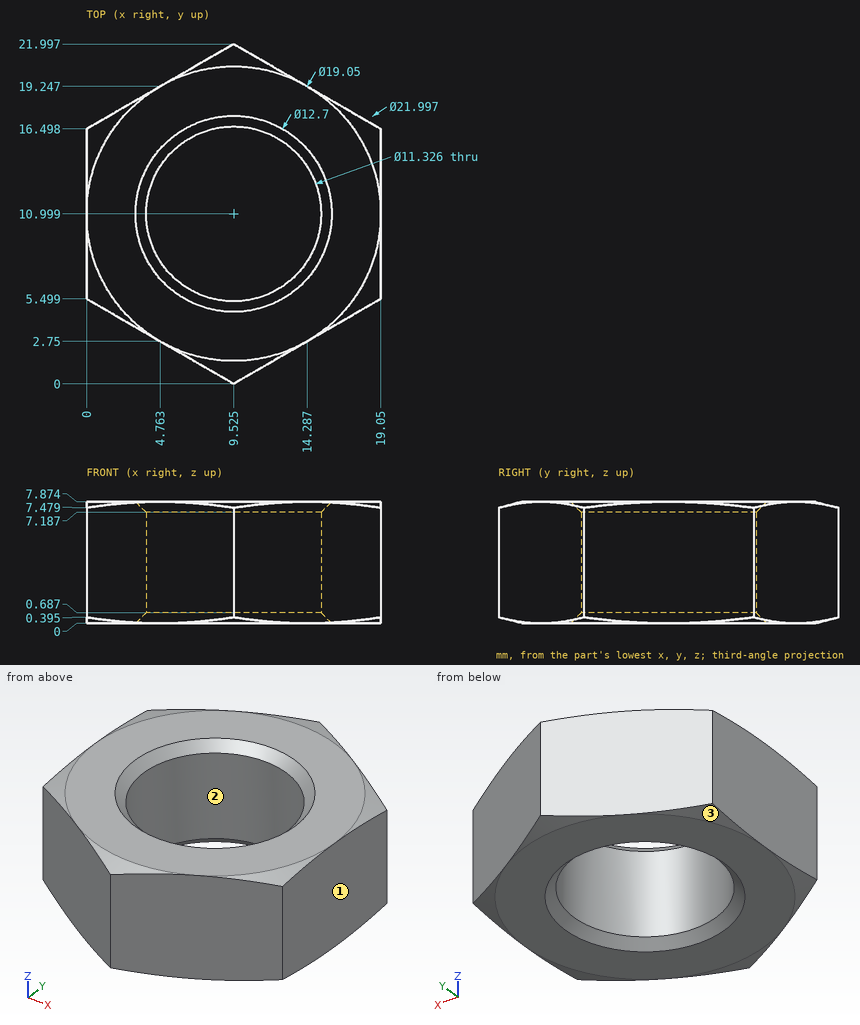
Design review of the part shown in the three views and the two pictorial views. Dimensions are in mm from the part's minimum x, y and z. Give positions to 0.01 mm unless a question says otherwise; leave off trailing zeros. Return JSON: item names as keys, results as strings. Group by question number.
(1) To check wall thickness, follow probe 1 along Y at (x, z) = (14.5, 6) (1 decimal); probe 2 along X at (y, z) = (12, 2); probe 3 along X at (y, z) = (7.5, 4). State the ranges of each line that lie inside material, in increasing order.
(2) Insertion check: pin 1 (4 mm diameter, centred on x = 6.5, z = 6, fed in from +Y) (1 decimal). The pin has a flat end and moves straight along its axis. Give the tip position at first contact, or say it passes through.
(3) Mouldability with a two-part tool opening along X and no side actions: class the marked faces 1, 2 and 3 as +X half, -X half, draft (parallel to the pull), parting line (faces both ways), or undercut.
Reported:
{
 "1": {"probe 1": "y = 2.9 to 8.3, 13.7 to 19.1", "probe 2": "x = 0 to 3.95, 15.1 to 19.05", "probe 3": "x = 0 to 5.07, 13.98 to 19.05"},
 "2": {"pin 1": "stops at y = 21.4"},
 "3": {"face 1": "+X half", "face 2": "undercut", "face 3": "-X half"}
}
